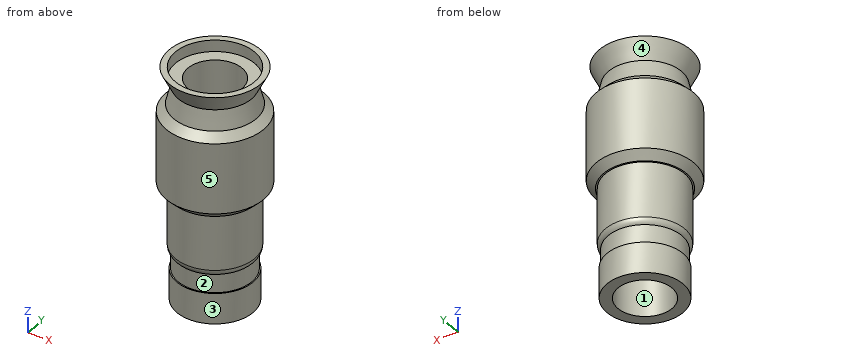
Autodesk Inventor part; units mm, degrees
ref_plane "Work Plane2" through (0, 0, 96.52) normal (0, 0, 1) x (1, 0, 0)
ref_plane "YZ Plane" through (0, 0, 0) normal (1, 0, 0) x (0, 1, 0)
ref_plane "XZ Plane" through (0, 0, 0) normal (0, 1, 0) x (-1, 0, 0)
sketch "Sketch1" plane through (0, 0, 0) normal (0, 0, 1) x (1, 0, 0)
  circle A0 centre (0, 0) radius 15.875
  dimension "d0" = 31.75
extrude "Extrusion1" add sketch "Sketch1" along normal blind 20.32
sketch "Sketch2" plane through (0, 0, 20.32) normal (0, 0, 1) x (1, 0, 0)
  circle A0 centre (0, 0) radius 15.367
  circle A1 centre (0, 0) radius 16.7085
  dimension "d5" = 30.734
extrude "Extrusion2" cut sketch "Sketch2" against normal blind 7.62
sketch "Sketch3" plane through (0, 0, 20.32) normal (0, 0, 1) x (1, 0, 0)
  circle A0 centre (0, 0) radius 16.51
  dimension "d6" = 33.02
extrude "Extrusion3" add sketch "Sketch3" along normal blind 25.4
fillet "Fillet1" radius 3.175 1 edges at (-16.51, 0, 20.32)
sketch "Sketch4" plane through (0, 0, 45.72) normal (0, 0, 1) x (1, 0, 0)
  circle A0 centre (0, 0) radius 20.32
  dimension "d10" = 40.64
extrude "Extrusion4" add sketch "Sketch4" along normal blind 35.56
chamfer "Chamfer1" distance 3.175 angle 45 2 edges at (-20.32, 0, 45.72) (-20.32, 0, 81.28)
sketch "Sketch5" plane through (0, 0, 0) normal (0, 1, 0) x (-1, 0, 0)
  point P0 (0, 0)
ref_plane "Work Plane1" through (0, 0, 88.9) normal (0, 0, 1) x (1, 0, 0)
sketch "Sketch6" plane through (0, 0, 88.9) normal (0, 0, 1) x (1, 0, 0)
  circle A0 centre (0, 0) radius 15.24
  dimension "d17" = 30.48
loft "Loft1" add profiles "Sketch6" section 1 edges at (-17.145, 0, 81.28)
ref_plane "Work Plane2" through (0, 0, 96.52) normal (0, 0, 1) x (1, 0, 0)
sketch "Sketch7" plane through (0, 0, 96.52) normal (0, 0, 1) x (1, 0, 0)
  circle A0 centre (0, 0) radius 19.05
  dimension "d23" = 38.1
loft "Loft2" add profiles "Sketch7" section 1 edges at (-15.24, 0, 88.9)
sketch "Sketch8" plane through (0, 0, 96.52) normal (0, 0, 1) x (1, 0, 0)
  circle A0 centre (0, 0) radius 16.51
extrude "Extrusion5" cut sketch "Sketch8" against normal blind 4.7625
sketch "Sketch9" plane through (0, 0, 91.7575) normal (0, 0, 1) x (1, 0, 0)
  circle A0 centre (0, 0) radius 11.2811
extrude "Extrusion6" cut sketch "Sketch9" against normal blind 120.65
properties part number "okular" material "Iron, Cast"
Source: CAD feature listing. Evaluate the final solid. Frame: model axes, mm. Face numbers are marked on the shaded views. A direction names the side the tool comes from. Give positions to 0.01 mm unless a question says otherwise; leave off trailing zeros. Loops run counter-clockwise (first coordinate to the right, second up) from the corner with the lowest first, then second, coordinate; pieces in that order, holes last. Notation, with made-up numbers: (5, 56) -> (23, 56) arc R22 ccw to (23, 87) -> close; hole circle Ø9 at (19, 46.5). An arc over 180 degrees is marked (long way). Put each result on its own line as item: value. Start each with the question number.
1) Cut plane C-C (z = 52.5). Return loops of the section in (x, y).
2) Material intervals for probe 1 along Y at (x, z) = (-0.5, 31.5); probe 2 along Z at (x, y) = (11, -5); probe 3 along Y at (x, z) = (-7, 47), sorted ascending.
3) Cut plane B-B (z = 87.5). Return loops of the section in (x, y), then the cut area to 3 significant figures.
4) Draft query along X for the marked faces 1 and 2. Return one class per face: released by +X, released by -X, zero draft, split by the parting line, or undercut.
5) Contact query for flat-ended pins moving along their axis: P1, Ø12, axis at y = -4, z = 25, coming from the +X side; P2, Ø8, axis at y = -15.5, z = 81, coming from the -X side; P3, Ø16, axis at x = -7.5, y = 2, coming from the +Z side. Output: stop coordinate, or through.
6) Reachability of the marked faces 3, 4 and 5 from +Z, -Z, +X, -X, +Y, -Y: full face, straight path, thin tool, end or side. Return the list, or none.
Results are:
1. outline: circle Ø40.64 at (0, 0); hole circle Ø22.56 at (0, 0)
2. probe 1: y = -16.5 to -11.27, 11.27 to 16.5
2. probe 2: z = 0 to 91.76
2. probe 3: y = -17.04 to -8.85, 8.85 to 17.04
3. outline: circle Ø31.18 at (0, 0); hole circle Ø22.56 at (0, 0)
3. area: 364 mm2
4. face 1: undercut
4. face 2: split by the parting line
5. P1: stops at x = 16.51
5. P2: stops at x = -15.83
5. P3: stops at z = 91.76
6. face 3: -Z
6. face 4: none
6. face 5: +Z, -Z
